```python
from build123d import *

# Parameters (mm, degrees)
SKETCH1_W           = 268.862640616
SKETCH1_H           = 111.719179434
BOSS_EXTRUDE1_DEPTH = 20
SKETCH2_W           = 210.712226585
SKETCH2_H           = 111.719179434
BOSS_EXTRUDE2_DEPTH = 20
SKETCH3_W           = 146.860036711
SKETCH3_H           = 111.719179434
BOSS_EXTRUDE3_DEPTH = 20
SKETCH5_W           = 87.947337462
SKETCH5_H           = 111.719179434
BOSS_EXTRUDE5_DEPTH = 20
SKETCH9_R           = 8.750978852
SKETCH9_R_2         = 8.685098526
CUT_EXTRUDE3_DEPTH  = 163.837867161
CUT_EXTRUDE4_DEPTH  = 177.963756124


with BuildPart() as part:
    # Sketch1 → Boss-Extrude1 (new body)
    with BuildSketch(Plane(origin=(0, 0, 0), x_dir=(1, 0, 0), z_dir=(0, 1, 0))):
        with Locations((12.89067455, -0.818455527)):
            Rectangle(SKETCH1_W, SKETCH1_H)
    extrude(amount=BOSS_EXTRUDE1_DEPTH)

    # Sketch2 → Boss-Extrude2 (add)
    with BuildSketch(Plane(origin=(0, 20, 0), x_dir=(1, 0, 0), z_dir=(0, 1, 0))):
        with Locations((12.379125057, -0.818455527)):
            Rectangle(SKETCH2_W, SKETCH2_H)
    extrude(amount=BOSS_EXTRUDE2_DEPTH)

    # Sketch3 → Boss-Extrude3 (add)
    with BuildSketch(Plane(origin=(0, 40, 0), x_dir=(1, 0, 0), z_dir=(0, 1, 0))):
        with Locations((10.905612982, -0.818455527)):
            Rectangle(SKETCH3_W, SKETCH3_H)
    extrude(amount=BOSS_EXTRUDE3_DEPTH)

    # Sketch5 → Boss-Extrude5 (add)
    with BuildSketch(Plane(origin=(0, 60, 0), x_dir=(1, 0, 0), z_dir=(0, 1, 0))):
        with Locations((12.234351136, -0.818455527)):
            Rectangle(SKETCH5_W, SKETCH5_H)
    extrude(amount=BOSS_EXTRUDE5_DEPTH)

    # Sketch9 → Cut-Extrude3 (cut, through all)
    with BuildSketch(Plane(origin=(0, 40, 0), x_dir=(1, 0, 0), z_dir=(0, 1, 0))):
        with Locations(Location((-78.994603396, 2.900710485, 0), (0, 0, 270))):
            Circle(SKETCH9_R)
        with Locations(Location((99.525365185, 2.900710485, 0), (0, 0, 270))):
            Circle(SKETCH9_R_2)
    extrude(amount=-CUT_EXTRUDE3_DEPTH, mode=Mode.SUBTRACT)

    # Sketch10 → Cut-Extrude4 (cut, through all)
    with BuildSketch(Plane(origin=(0, 80, 0), x_dir=(1, 0, 0), z_dir=(0, 1, 0))):
        Polygon((23.264076608, -31.015956355), (39.082685924, -10.377494547), (29.11855836, 13.641053878), (3.335821481, 17.021140493), (-12.482787835, -3.617321315), (-2.518660272, -27.63586974), align=None)
    extrude(amount=-CUT_EXTRUDE4_DEPTH, mode=Mode.SUBTRACT)


solid = part.part
```
Input: part model. Units: mm. Frame: model coordinates. A direction names the side the tool comes from. Coordinates: 2 decimals unless noted, no trailing zeros. Write each loop counter-clockwise with the first axis right and the second up, starting at its lowest first coordinate (ties: lowest second). Pieces come first, ordered by that corner, then holes. Notation, with made-up numbers: M 43,4.5 L 59,4.5 A19 ccw 59,12.5 Z; hole C 3,-24 d1. An arc over 180 degrees is marked long. Use one line per item in the form item = value.
Q1. Section B-B (z = 24.5). Return loops of the section in (x, y), plus the area to 3 significant figures.
Answer below:
outline = M -121.54,0 L -3.82,0 L -3.82,80 L -31.74,80 L -31.74,60 L -62.52,60 L -62.52,40 L -92.98,40 L -92.98,20 L -121.54,20 Z; M 28.26,0 L 147.32,0 L 147.32,20 L 117.74,20 L 117.74,40 L 84.34,40 L 84.34,60 L 56.21,60 L 56.21,80 L 28.26,80 Z
area = 11,700 mm²
Q2. Section C-C (x = 36.5). Return loops of the section in (y, z).
Answer below:
outline = M 0,-55.04 L 80,-55.04 L 80,4.15 L 0,4.15 Z; M 0,13.75 L 80,13.75 L 80,56.68 L 0,56.68 Z
Q3. Draft query along X for faces 4 (the face through (-88, 40, 0)), 5 (the face through (-7.57, 40.56, 15.46)), 6 (the face through (-31.739, 70, 2)). Return one class per face: released by +X, released by -X, zero draft, split by the parting line, or undercut.
Answer below:
face_4 = zero draft
face_5 = undercut
face_6 = released by -X
Q4. Material intervals for probe 1 along Y at (x, z) = (78.5, 19); probe 2 along X at (y, z) = (26.5, 26); probe 3 along Z at (x, y) = (14, 37.5), sorted ascending. Write a range as from..to.
Answer below:
probe_1 = 0..60
probe_2 = -92.98..-3.2, 27.11..117.74
probe_3 = -55.04..-15.62, 29.8..56.68
Q5. Set-up query: faces 1 (the face through (10.19, 40.56, 29.3)), 2 (the face through (70, 60, 0)), 3 (the face through (-47, 60, 0)). Return all of +Z, -Z, +X, -X, +Y, -Y with unobstructed straight access to the full face (end or side cutting, diameter ignored); none if empty.
Answer below:
face_1 = +Y, -Y
face_2 = +Z, -Z, +X, +Y
face_3 = +Z, -Z, -X, +Y
Q6. Section A-A (y = 43.5). Return loops of the section in (x, z), plus the area to 3 significant figures.
Answer below:
outline = M -62.52,-55.04 L 84.34,-55.04 L 84.34,56.68 L -62.52,56.68 Z; hole M -12.48,3.62 L 3.34,-17.02 L 29.12,-13.64 L 39.08,10.38 L 23.26,31.02 L -2.52,27.64 Z
area = 14,700 mm²
Q7. Section D-D (z = 1). Return loops of the section in (x, y).
Answer below:
outline = M -121.54,0 L -86.83,0 L -86.83,40 L -92.98,40 L -92.98,20 L -121.54,20 Z; M -71.16,0 L -10.48,0 L -10.48,80 L -31.74,80 L -31.74,60 L -62.52,60 L -62.52,40 L -71.16,40 Z; M 35.19,0 L 91.77,0 L 91.77,40 L 84.34,40 L 84.34,60 L 56.21,60 L 56.21,80 L 35.19,80 Z; M 107.29,0 L 147.32,0 L 147.32,20 L 117.74,20 L 117.74,40 L 107.29,40 Z
Q8. First-contact query: pin 1 (16 mm diameter, centred on x = -78.99, z = -2.9, fed in from -Y); pin 2 (6 mm diameter, centred on x = -94, z = 42, fed in from +Y); pin 3 (10 mm diameter, centred on y = 66.5, z = 28.5, fed in from +X); pin 4 (5 mm diameter, centred on y = 39.5, z = -25.5, fed in from +X). Flat tips, straight axial feed; report the tip coordinate or a pass-through.
Answer below:
pin_1 = through
pin_2 = 40
pin_3 = 56.21
pin_4 = 117.74
